from build123d import *

# Parameters (mm, degrees)
F0_R     = 4.1275
F1_DEPTH = 3.175
F2_R     = 5.08


with BuildPart() as f1:
    # F0 (on Top) → F1 (new body)
    with BuildSketch(Plane.XY):
        Polygon((15.875, 77.233556), (-15.875, 77.233556), (-15.875, -49.766444), (-41.275, -49.766444), (-41.275, -75.166444), (15.875, -75.166444), align=None)
        with Locations((0, -49.766444)):
            Circle(F0_R, mode=Mode.SUBTRACT)
        with Locations((0, 51.833556)):
            Circle(F0_R, mode=Mode.SUBTRACT)
    extrude(amount=F1_DEPTH)

    # F2
    f2_edges = [f1.edges().sort_by_distance(p)[0] for p in [
        (-15.875, 77.233556, 1.5875),
        (15.875, 77.233556, 1.5875),
        (-15.875, -49.766444, 1.5875),
        (-41.275, -49.766444, 1.5875),
        (-41.275, -75.166444, 1.5875),
        (15.875, -75.166444, 1.5875),
    ]]
    fillet(f2_edges, radius=F2_R)


solid = f1.part
Geometry check sheet. Reference: the model listing, model coordinates, mm. A direction names the side the tool comes from. Coordinates: 2 decimals unless noted, no trailing zeros. Write each loop counter-clockwise with the first axis right and the second up, starting at its lowest first coordinate (ties: lowest second). Pieces come first, ordered by that corner, then holes. Notation, with made-up numbers: (40, -32) -> (68, -32) arc R17 ccw to (68, -15) -> close; hole circle Ø5 at (23, 45). An arc over 180 degrees is marked (long way). One line per question, with ' | ' between items.
1. Thickness scan on probe 1 along Y at (x, z) = (0, 2.5); probe 2 along Y at (x, z) = (1.5, 1.7); probe 3 along Y at (x, z) = (-24.5, 1.55). Record the ranges inside material, lowest first. Write a range as from..to.
Answers:
probe 1: y = -75.17..-53.89, -45.64..47.71, 55.96..77.23 | probe 2: y = -75.17..-53.61, -45.92..47.99, 55.68..77.23 | probe 3: y = -75.17..-49.77
2. Cross-section at D-D on x = -17.5. Record the cut outline in (y, z) (3 decimals).
Answers:
outline: (-75.166, 0) -> (-48.411, 0) -> (-48.411, 3.175) -> (-75.166, 3.175) -> close
3. Set-up check for faces 4 (the flat face through (-28, -49.766, 2)), 5 (the flat face through (0, 2, 3.175)): record each of +Z, -Z, +X, -X, +Y, -Y from which the full face is reachable in a straight line by a thin tool's end or side.
Answers:
face 4: +Z, -Z, -X, +Y | face 5: +Z, +X, -X, +Y, -Y
4. Cross-section at C-C on y = -22. Record the cut outline in (x, z) (3 decimals), and give its area (3 significant figures).
Answers:
outline: (-15.875, 0) -> (15.875, 0) -> (15.875, 3.175) -> (-15.875, 3.175) -> close | area: 101 mm²
5. Cross-section at B-B on z = 2.25. Record the cut outline in (x, y) (1 decimal), and give its area (3 significant figures).
Answers:
outline: (-41.3, -70.1) arc R5.1 ccw to (-36.2, -75.2) -> (10.8, -75.2) arc R5.1 ccw to (15.9, -70.1) -> (15.9, 72.2) arc R5.1 ccw to (10.8, 77.2) -> (-10.8, 77.2) arc R5.1 ccw to (-15.9, 72.2) -> (-15.9, -44.7) arc R5.1 cw to (-21, -49.8) -> (-36.2, -49.8) arc R5.1 ccw to (-41.3, -54.8) -> close; hole circle Ø8.3 at (0, -49.8); hole circle Ø8.3 at (0, 51.8) | area: 5,350 mm²
6. Depth check by flat-ended pin: pin 1 Ø5 at (x, y) = (0, 51.83) entering from +Z; pin 2 Ø1.6 at (y, z) = (-4.5, 1.5) entering from -X (3 decimals). Enter the tip coordinate at first touch or a pass-through.
Answers:
pin 1: passes through | pin 2: stops at x = -15.875
7. Cross-section at A-A on x = 0. Record the cut outline in (y, z) (3 decimals).
Answers:
outline: (-75.166, 0) -> (-53.894, 0) -> (-53.894, 3.175) -> (-75.166, 3.175) -> close; (-45.639, 0) -> (47.706, 0) -> (47.706, 3.175) -> (-45.639, 3.175) -> close; (55.961, 0) -> (77.234, 0) -> (77.234, 3.175) -> (55.961, 3.175) -> close
8. Draft check along Y on faces 1 (the cylindrical face through (14.426, -73.639, 1.61)), 2 (the cylindrical face through (1.9, 48.17, 1.57)), 3 (the cylindrical face through (-14.35, 75.78, 1.61)). Enter one of: +Y half, -Y half, draft (parallel to the pull), parting line (faces both ways), or undercut.
Answers:
face 1: -Y half | face 2: undercut | face 3: +Y half
